```python
from build123d import *

# Parameters (mm, degrees)
SKETCH1_W           = 15.6
SKETCH1_H           = 15.6
BOSS_EXTRUDE1_DEPTH = 5
BOSS_EXTRUDE2_DEPTH = 7.8
BOSS_EXTRUDE3_DEPTH = 4.05
SKETCH4_R           = 1.925
BOSS_EXTRUDE4_DEPTH = 3
SKETCH6_R           = 0.65
BOSS_EXTRUDE5_DEPTH = 4


with BuildPart() as part:
    # Sketch1 → Boss-Extrude1 (new body)
    with BuildSketch(Plane(origin=(0, 0, 0), x_dir=(1, 0, 0), z_dir=(0, 1, 0))):
        Rectangle(SKETCH1_W, SKETCH1_H)
    extrude(amount=BOSS_EXTRUDE1_DEPTH)

    # Sketch2 → Boss-Extrude2 (add, symmetric)
    with BuildSketch(Plane(origin=(0, 0, 0), x_dir=(0, 0, -1), z_dir=(1, 0, 0))):
        Polygon((-7.8, 5), (7.8, 5), (6.918365096, 10), (-4.913248654, 10), align=None)
    extrude(amount=BOSS_EXTRUDE2_DEPTH, both=True)

    # Sketch3 → Boss-Extrude3 (add)
    with BuildSketch(Plane(origin=(0, 10, 0), x_dir=(1, 0, 0), z_dir=(0, 1, 0))):
        Polygon((-0.65, 2), (0.65, 2), (0.65, 0.65), (2, 0.65), (2, -0.65), (0.65, -0.65), (0.65, -2), (-0.65, -2), (-0.65, -0.65), (-2, -0.65), (-2, 0.65), (-0.65, 0.65), align=None)
    extrude(amount=BOSS_EXTRUDE3_DEPTH)

    # Sketch4 → Boss-Extrude4 (add)
    with BuildSketch(Plane(origin=(0, 0, 0), x_dir=(1, 0, 0), z_dir=(0, 1, 0))):
        with Locations(Location((0, 0, 0), (0, 0, 270))):
            Circle(SKETCH4_R)
    extrude(amount=-BOSS_EXTRUDE4_DEPTH)

    # Sketch6 → Boss-Extrude5 (add)
    with BuildSketch(Plane(origin=(0, 0, 0), x_dir=(1, 0, 0), z_dir=(0, 1, 0))):
        with Locations(Location((2.54, 5.08, 0), (0, 0, 270))):
            Circle(SKETCH6_R)
        with Locations(Location((-3.81, 2.54, 0), (0, 0, 270))):
            Circle(SKETCH6_R)
    extrude(amount=-BOSS_EXTRUDE5_DEPTH)


solid = part.part
```
Verification items for the finished model (mm, model axes). A direction names the side the tool comes from. Coordinates: 2 decimals unless noted, no trailing zeros. Write each loop counter-clockwise with the first axis right and the second up, starting at its lowest first coordinate (ties: lowest second). Pieces come first, ordered by that corner, then holes. Notation, with made-up numbers: (81.5, 64.25) - (131.5, 64.25) arc R19 cw to (131.5, 97.25) - close; hole circle Ø11 at (68.25, 75.5). An arc over 180 degrees is marked (long way). Write item = value, one per line.
Q1. Go/stop test with flat-tipped pins: pin 1 Ø1.4 at (y, z) = (12, -0.5) entering from +X; pin 2 Ø1.1 at (x, y) = (-1, 12) entering from +Z; pin 3 Ø1.1 at (y, z) = (11.5, -1.5) entering from +X. Record where each tip stops, or that it passes through.
Answer:
pin_1 = 2
pin_2 = 2
pin_3 = 0.65
Q2. Cross-section at A-A (x = 0). Enter the section's corners in (y, z) (3 decimals).
Answer:
outline = (-3, -1.925) - (0, -1.925) - (0, -7.8) - (5, -7.8) - (10, -6.918) - (10, -2) - (14.05, -2) - (14.05, 2) - (10, 2) - (10, 4.913) - (5, 7.8) - (0, 7.8) - (0, 1.925) - (-3, 1.925) - close
Q3. Cross-section at B-B (z = 0). Enter the section's corners in (x, y) (3 decimals), plus the area to 3 significant figures.
Answer:
outline = (-7.8, 0) - (-1.925, 0) - (-1.925, -3) - (1.925, -3) - (1.925, 0) - (7.8, 0) - (7.8, 10) - (2, 10) - (2, 14.05) - (-2, 14.05) - (-2, 10) - (-7.8, 10) - close
area = 184 mm²
Q4. Access from +Z, -Z, +X, -X, +Y, -Y to the whole of each face (thin tool, end or side, straight path). Record for faces 1 (the face through (0.65, 12, -1)), 2 (the face through (2.74, -1.97, -4.46)), 3 (the face through (0.65, 12, 1)), 4 (the face through (0, 12, 2)).
Answer:
face_1 = -Z, +X, +Y
face_2 = -Y
face_3 = +Z, +X, +Y
face_4 = +Z, +X, -X, +Y
Q5. Material ranges on L1, parallel to Y at x = 0, z = -0.5; L2, parallel to Y at x = 4.5, z = 2; L3, parallel to Z at x = -1.25, y = 11.25, recorded low to high. Write a range as from..to.
Answer:
L1 = -3..14.05
L2 = 0..10
L3 = -0.65..0.65
Q6. Cross-section at D-D (x = 4.75). Enter the section's corners in (y, z), plus the area to 3 significant figures.
Answer:
outline = (0, -7.8) - (5, -7.8) - (10, -6.92) - (10, 4.91) - (5, 7.8) - (0, 7.8) - close
area = 147 mm²
Q7. Cross-section at C-C (z = -2.54). Enter the section's corners in (x, y).
Answer:
outline = (-7.8, 0) - (-4.46, 0) - (-4.46, -4) - (-3.16, -4) - (-3.16, 0) - (7.8, 0) - (7.8, 10) - (-7.8, 10) - close
